```python
from build123d import *

# Parameters (mm, degrees)
F1_DEPTH = 9.525
F2_D     = 5
F3_R     = 2.54
F4_DEPTH = 4.7


# Not quite as in the source:
# - a feature names something its author has since deleted; it is built from what else it names


with BuildPart() as f1:
    # F0 (on Top) → F1 (new body)
    with BuildSketch(Plane.XY):
        with BuildLine():
            Line((25.4, 29.2563221224), (-25.4, 29.2563221224))
            ThreePointArc((-25.4, 29.2563221224), (-34.925, 19.7313221224), (-25.4, 10.2063221224))
            Line((-25.4, 10.2063221224), (-22.225, 10.2063221224))
            ThreePointArc((-22.225, 10.2063221224), (-13.2447438789, 6.4865782435), (-9.525, -2.4936778776))
            Line((-9.525, -2.4936778776), (-9.525, -42.2686778776))
            ThreePointArc((-9.525, -42.2686778776), (0, -51.7936778776), (9.525, -42.2686778776))
            Line((9.525, -42.2686778776), (9.525, -2.4936778776))
            ThreePointArc((9.525, -2.4936778776), (13.2447438789, 6.4865782435), (22.225, 10.2063221224))
            Line((22.225, 10.2063221224), (25.4, 10.2063221224))
            ThreePointArc((25.4, 10.2063221224), (34.925, 19.7313221224), (25.4, 29.2563221224))
        make_face()
        Polygon((-4.9074772881, -42.2686778776), (-2.4537386441, -38.0186778776), (2.4537386441, -38.0186778776), (4.9074772881, -42.2686778776), (2.4537386441, -46.5186778776), (-2.4537386441, -46.5186778776), align=None, mode=Mode.SUBTRACT)
        Polygon((-20.4925227119, 19.7313221224), (-22.9462613559, 15.4813221224), (-27.8537386441, 15.4813221224), (-30.3074772881, 19.7313221224), (-27.8537386441, 23.9813221224), (-22.9462613559, 23.9813221224), align=None, mode=Mode.SUBTRACT)
        Polygon((30.3074772881, 19.7313221224), (27.8537386441, 15.4813221224), (22.9462613559, 15.4813221224), (20.4925227119, 19.7313221224), (22.9462613559, 23.9813221224), (27.8537386441, 23.9813221224), align=None, mode=Mode.SUBTRACT)
        Polygon((2.4537386441, -38.0186778776), (-2.4537386441, -38.0186778776), (-4.9074772881, -42.2686778776), (-2.4537386441, -46.5186778776), (2.4537386441, -46.5186778776), (4.9074772881, -42.2686778776), align=None)
        Polygon((-27.8537386441, 15.4813221224), (-22.9462613559, 15.4813221224), (-20.4925227119, 19.7313221224), (-22.9462613559, 23.9813221224), (-27.8537386441, 23.9813221224), (-30.3074772881, 19.7313221224), align=None)
        Polygon((22.9462613559, 15.4813221224), (27.8537386441, 15.4813221224), (30.3074772881, 19.7313221224), (27.8537386441, 23.9813221224), (22.9462613559, 23.9813221224), (20.4925227119, 19.7313221224), align=None)
    extrude(amount=F1_DEPTH)

    # F2 (through all)
    with Locations(Plane(origin=(0, 0, 0), x_dir=(1, 0, 0), z_dir=(0, 0, -1))):
        with Locations((25.4, -19.7313221224), (-25.4, -19.7313221224), (0, 42.2686778776)):
            Hole(F2_D / 2)

    # F3
    f3_edges = [f1.edges().sort_by_distance(p)[0] for p in [
        (0, 29.256322, 0),
        (0, 29.256322, 9.525),
    ]]
    fillet(f3_edges, radius=F3_R)

    # F0 (on Top) → F4 (cut)
    with BuildSketch(Plane.XY):
        Polygon((2.4537386441, -38.0186778776), (-2.4537386441, -38.0186778776), (-4.9074772881, -42.2686778776), (-2.4537386441, -46.5186778776), (2.4537386441, -46.5186778776), (4.9074772881, -42.2686778776), align=None)
        Polygon((-27.8537386441, 15.4813221224), (-22.9462613559, 15.4813221224), (-20.4925227119, 19.7313221224), (-22.9462613559, 23.9813221224), (-27.8537386441, 23.9813221224), (-30.3074772881, 19.7313221224), align=None)
        Polygon((22.9462613559, 15.4813221224), (27.8537386441, 15.4813221224), (30.3074772881, 19.7313221224), (27.8537386441, 23.9813221224), (22.9462613559, 23.9813221224), (20.4925227119, 19.7313221224), align=None)
    extrude(amount=F4_DEPTH, mode=Mode.SUBTRACT)


solid = f1.part
```
CAD build for the part. Positions are in the model's coordinates, mm. A direction names the side the tool comes from. Round coordinates to 2 decimals unless told otherwise and drop trailing zeros. Write each loop counter-clockwise with the first axis right and the second up, starting at its lowest first coordinate (ties: lowest second). Pieces come first, ordered by that corner, then holes. Notation, with made-up numbers: M -11.5,62 L 21.5,62 A22 ccw 21.5,84 Z; hole C -31.5,-3.75 d9. An arc over 180 degrees is marked long. One line per question, with ' | ' between items.
1. Probe L1, parallel to Y at x = 0, z = 5.75; L2, parallel to X at y = 21, z = 8.5; L3, parallel to X at y = -25, z = 4 (3 decimals). List the from-to ranges inside material, lowest first. Write a range as from..to.
Working result:
L1: -51.79..-44.77, -39.77..29.26 | L2: -34.33..-27.55, -23.25..23.25, 27.55..34.33 | L3: -9.525..9.525
2. Cut at B-B on z = 1. Write the cut outline in (x, y) (3 decimals), and give its area (3 significant figures).
Working result:
outline: M -25.4,10.726 L -22.225,10.726 A13.22 cw -9.005,-2.494 L -9.005,-42.269 A9.005 ccw 9.005,-42.269 L 9.005,-2.494 A13.22 cw 22.225,10.726 L 25.4,10.726 A9.005 ccw 25.4,28.736 L -25.4,28.736 A9.005 ccw Z; hole M -30.307,19.731 L -27.854,15.481 L -22.946,15.481 L -20.493,19.731 L -22.946,23.981 L -27.854,23.981 Z; hole M -4.907,-42.269 L -2.454,-46.519 L 2.454,-46.519 L 4.907,-42.269 L 2.454,-38.019 L -2.454,-38.019 Z; hole M 20.493,19.731 L 22.946,15.481 L 27.854,15.481 L 30.307,19.731 L 27.854,23.981 L 22.946,23.981 Z | area: 2,140 mm2
3. Cut at A-A on x = 0. Write the cut outline in (y, z) (3 decimals), and give its area (3 significant figures).
Working result:
outline: M -51.794,2.54 A2.54 ccw -49.254,0 L -46.519,0 L -46.519,4.7 L -44.769,4.7 L -44.769,9.525 L -49.254,9.525 A2.54 ccw -51.794,6.985 Z; M -39.769,4.7 L -38.019,4.7 L -38.019,0 L 26.716,0 A2.54 ccw 29.256,2.54 L 29.256,6.985 A2.54 ccw 26.716,9.525 L -39.769,9.525 Z | area: 702 mm2
4. Cut at C-C on y = -18. Write the cut outline in (x, z) (3 decimals), and give its area (3 significant figures).
Working result:
outline: M -9.525,2.54 A2.54 ccw -6.985,0 L 6.985,0 A2.54 ccw 9.525,2.54 L 9.525,6.985 A2.54 ccw 6.985,9.525 L -6.985,9.525 A2.54 ccw -9.525,6.985 Z | area: 176 mm2
5. Mould opens along X. For faces 5 (the flat face through (-21.702, 21.827, 2.317)), 6 (the flat face through (0, 6, 9.525)), 7 (the cylindrical face through (-27.71, 20.69, 7.15)), 8 (the cylindrical face through (-8.8, -22.66, 8.76)) say: pulls with the +X half, pulls with the -X half, needs draft (parallel to the pull), parting line crosses it, or undercut.
Working result:
face 5: undercut | face 6: needs draft | face 7: undercut | face 8: pulls with the -X half
6. Which spindle directions (+Z, -Z, +X, -X, +Y, -Y) get a long thin tool onto all of the face, cutting with end or side? Do faces 1 (the cylindrical face through (8.8, -22.1, 8.76)), 2 (the cylindrical face through (-8.801, -22.66, 0.764)), 3 (the flat face through (-21.737, 17.577, 2.317)), 4 (the cylindrical face through (-23.79, 10.93, 8.76)). Say none if no direction does.
Working result:
face 1: +Z, +X, -Y | face 2: -Z, -X, -Y | face 3: -Z | face 4: +Z, -X, -Y
7. Pin check, flat tips, straight feed: pin 1 Ø2 at (x, z) = (13, 7) entering from -Y; pin 2 Ø3.5 at (x, z) = (-23, 4.5) entering from -Y; pin 3 Ø2 at (y, z) = (-30.5, 4.5) entering from -X (3 decimals). Stop position of each tip, or through.
Working result:
pin 1: y = 5.04 | pin 2: y = 10.17 | pin 3: x = -9.525
